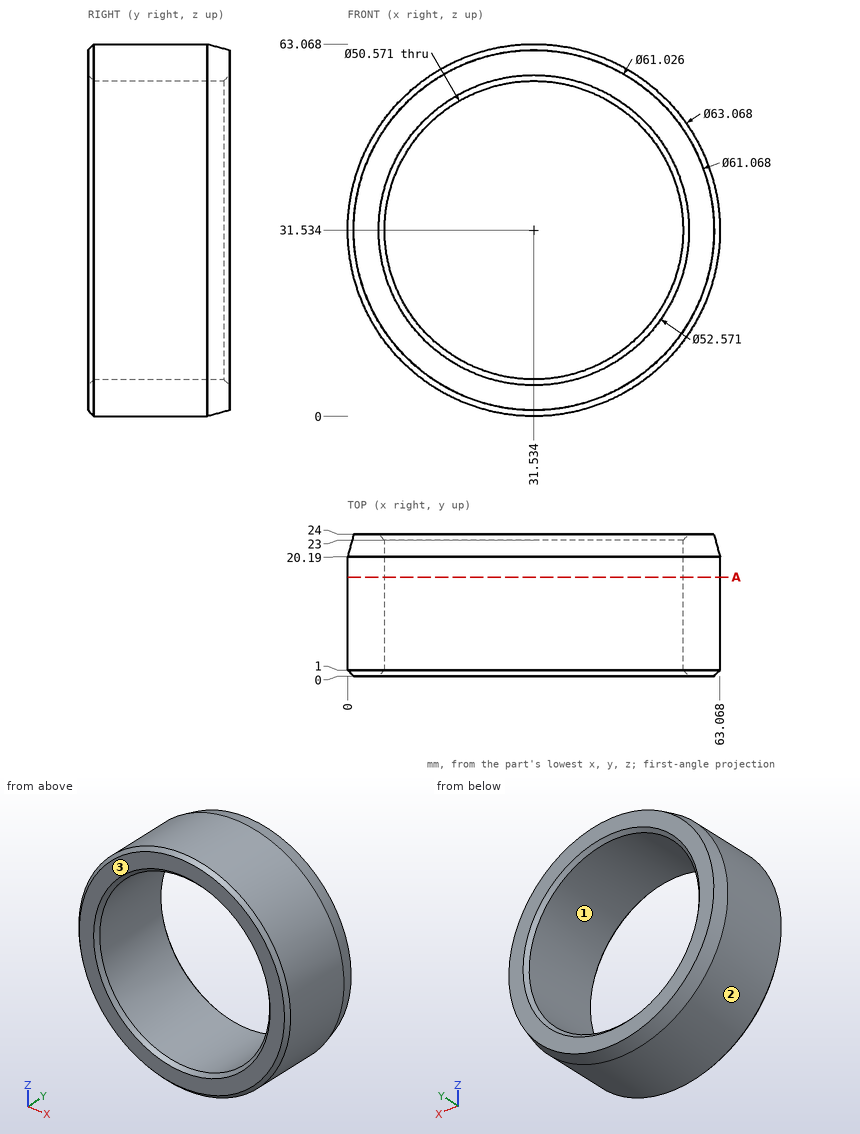
The drawing under review shows one solid part. Ordinate dimensions are in mm from its lowest x, y, z. Give positions to 0.01 mm unless a question says otherwise; leave off trailing zeros. Order: outer loops, then holes, each group sorted by start corner. A loop starts at its lowest first (then second) coordinate and runs counter-clockwise, first axis right, second up. Notation, with made-up numbers: (45, 83) -> (63, 83) arc R17 ccw to (63, 108) -> close; hole circle Ø4 at (71, -14.75). An arc over 180 degrees is marked (long way). Write item = value, one per line. Start each with the question number.
(1) To check wall thickness, follow line 1 along Z through (x, y) = (32, 8.5) (1 decimal); line 2 along Z through (x, y) = (30, 6.5) (1 decimal); line 3 along X through (y, z) = (12.5, 53.5) (1 decimal). State the ranges of each line that lie inside material, in increasing order.
(2) Mouldability with a two-part tool opening along X and no side actions: class the marked faces 1, 2 and 3 as +X half, -X half, draft (parallel to the pull), parting line (faces both ways), or undercut.
(3) For pin 1 (5 mm diameter, centred on x = 50.5, z = 41, fed in from +Y); pin 2 (5 mm diameter, centred on y = 6.5, z = 53, fed in from -X); pin 3 (6 mm diameter, centred on y = 16.5, z = 15, fed in from -X); pin 4 (3 mm diameter, centred on x = 29.5, y = 2.5, fed in from +Z), all flat-tipped, find the tip position at first contact; note any pin that passes through.
(4) We need section A-A on y = 16.75. Write out the cut boundary in (x, z) (1 decimal), plus the area to 3 significant figures.
Numbers:
q1.line_1 = 0 to 6.3, 56.8 to 63.1
q1.line_2 = 0 to 6.3, 56.8 to 63
q1.line_3 = 8.9 to 19, 44.1 to 54.2
q2.face_1 = undercut
q2.face_2 = parting line
q2.face_3 = draft
q3.pin_1 = through
q3.pin_2 = 6.34
q3.pin_3 = 3.05
q3.pin_4 = 63.06
q4.outline = circle Ø63.1 at (31.5, 31.5); hole circle Ø50.6 at (31.5, 31.5)
q4.area = 1,120 mm^2
